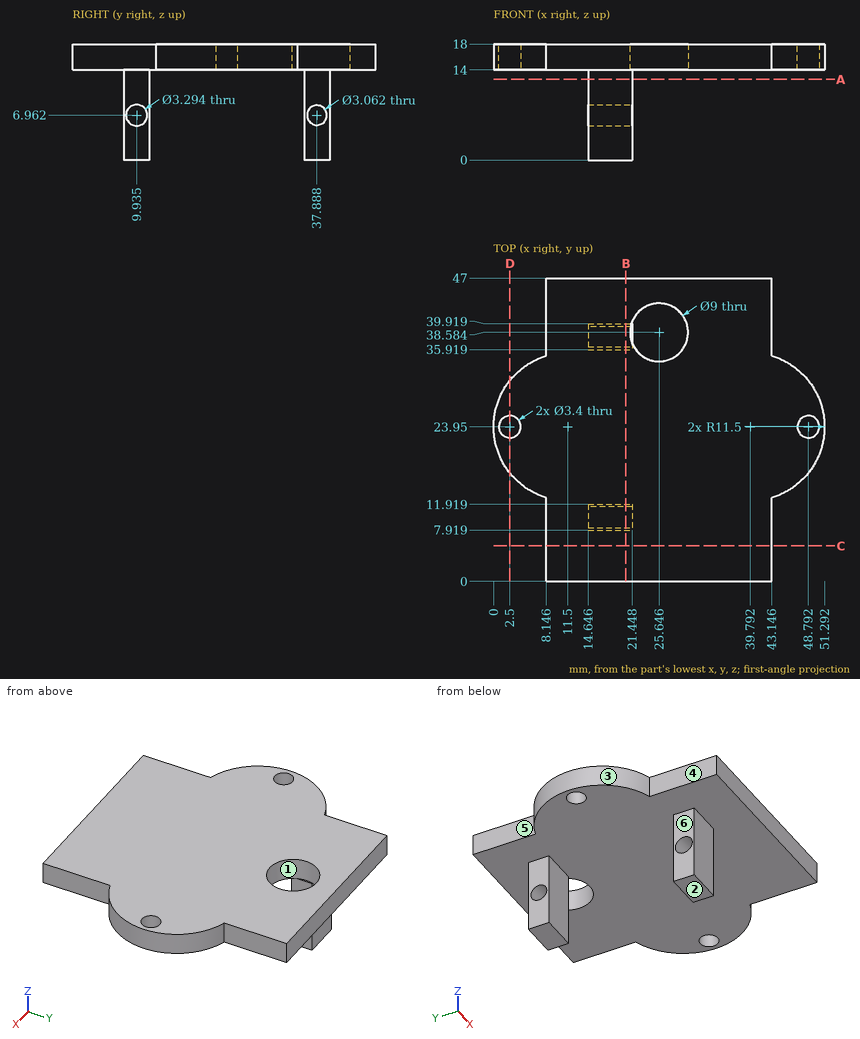
Geometry: see drawing. Coordinates: mm, zero at the bounding-box minimum. A direction names the side the tool comes from. Coordinates: 2 decimals unless noted, no trailing zeros. Loops run counter-clockwise (first coordinate to the right, second up) from the corner with the lowest first, then second, coordinate; pieces in that order, holes last.
(1) Material intervals for probe 1 along Z at (x, y) = (22.5, 27.5); probe 2 along Y at (x, z) = (2.5, 15.8); probe 3 along X at (y, z) = (34, 14.5) (1 decimal), sorted ascending.
(2) Pull-direction query (Y, two-part tool) for the marked faces 1, 2 and 3; classes: released by +Y, released by -Y, zero draft, split by the parting line, or undercut.
(3) Section C-C on y = 5.5. Return the cut outline in (x, z) (1 decimal), then the cut area to 3 significant figures.
(4) Section D-D on x = 2.5. Return the cut outline in (y, z).
(5) Section B-B on x = 20.5. Return the cut outline in (y, z) (1 decimal).
(6) Set-up query: the marked faces 4, 5 and 6. Return all of +Z, -Z, +X, -X, +Y, -Y with unobstructed straight access to the full face (end or side cutting, diameter ignored); none if empty.
(7) First-contact query: pin 1 Ø3 at (y, z) = (7.5, 16) entering from +X; pin 2 Ø1.2 at (y, z) = (9, 16) entering from -X; pin 3 Ø1.2 at (y, z) = (9.5, 5) entering from -X. Flat tips, straight axial feed; report the tip coordinate or a pass-through.
(8) Section A-A on z = 12.5. Return the cut outline in (x, y) (1 decimal).
Data:
1. probe 1: z = 14 to 18
1. probe 2: y = 16.79 to 22.25, 25.65 to 31.11
1. probe 3: x = 5.9 to 45.4
2. face 1: undercut
2. face 2: zero draft
2. face 3: split by the parting line
3. outline: (8.1, 14) - (43.1, 14) - (43.1, 18) - (8.1, 18) - close
3. area: 140 mm2
4. outline: (16.79, 14) - (22.25, 14) - (22.25, 18) - (16.79, 18) - close; (25.65, 14) - (31.11, 14) - (31.11, 18) - (25.65, 18) - close
5. outline: (0, 14) - (7.9, 14) - (7.9, 0) - (11.9, 0) - (11.9, 14) - (35.9, 14) - (35.9, 0) - (39.9, 0) - (39.9, 14) - (47, 14) - (47, 18) - (0, 18) - close; hole circle Ø3.3 at (9.9, 7); hole circle Ø3.1 at (37.9, 7)
6. face 4: +Z, -Z, -X, -Y
6. face 5: +Z, -Z, -X, +Y
6. face 6: -Z, -X, +Y, -Y
7. pin 1: stops at x = 43.15
7. pin 2: stops at x = 8.15
7. pin 3: stops at x = 14.65
8. outline: (14.6, 7.9) - (21.4, 7.9) - (21.4, 11.9) - (14.6, 11.9) - close; (14.6, 35.9) - (21.4, 35.9) - (21.4, 39.9) - (14.6, 39.9) - close
